Verification items for the finished model (mm, model axes). Give positions to 0.01 mm unless a question says otherwise; leave off trailing zeros. Order: outer loops, then holes, each group sorted by start corner. A loop starts at its lowest first (then second) coordinate and runs counter-clockwise, first axis right, second up.
(1) Sectioned sample at C-C on x = 76.2. Record the cut outline in (y, z) (3 decimals).
(2) Sectioned sample at B-B on z = 3.75. Count the separate pieces of the cut face and the enclosed holes in it, plus the area to 3 significant figures.
(3) Gauge pin test, flat end, axial feed: pin 1 (1 mm diameter, centred on y = -33, z = 4, fed in from +X). Record the tip position at first contact, or that the pin passes through.
(4) Sectioned sample at A-A on y = -32. Record the cut outline in (x, z), plus the area to 3 significant figures.
(5) Sectioned sample at D-D on y = -4.5. Record the cut outline in (x, z), plus the area to 3 significant figures.
(6) Scan lines: L1, parallel to Y at x = 0, z = 3; L2, parallel to X at y = -29.5, z = 4; L3, parallel to X at y = -9, z = 1. Record each from-to range of solid material in increasing order.
```python
from build123d import *

# Parameters (mm, degrees)
F0_R     = 1.5875
F1_DEPTH = 6.35


with BuildPart() as f1:
    # F0 (on Top) → F1 (new body)
    with BuildSketch(Plane.XY):
        with BuildLine():
            Line((152.4, 0), (0, 0))
            ThreePointArc((0, 0), (-19.05, -19.05), (0, -38.1))
            Line((0, -38.1), (60.325, -38.1))
            ThreePointArc((60.325, -38.1), (76.2, -22.225), (92.075, -38.1))
            Line((92.075, -38.1), (152.4, -38.1))
            ThreePointArc((152.4, -38.1), (171.45, -19.05), (152.4, 0))
        make_face()
        with Locations((0, -28.575)):
            Circle(F0_R, mode=Mode.SUBTRACT)
        with Locations((152.4, -28.575)):
            Circle(F0_R, mode=Mode.SUBTRACT)
        with Locations((0, -9.525)):
            Circle(F0_R, mode=Mode.SUBTRACT)
        with Locations((152.4, -9.525)):
            Circle(F0_R, mode=Mode.SUBTRACT)
    extrude(amount=F1_DEPTH)


solid = f1.part
```
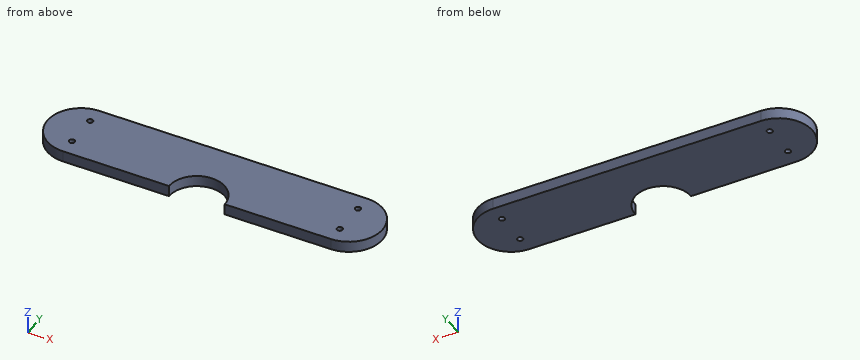
Ans:
1. outline: (-22.225, 0) - (0, 0) - (0, 6.35) - (-22.225, 6.35) - close
2. separate pieces: 1
2. enclosed holes: 4
2. area: 6,520 mm2
3. pin 1: stops at x = 165.89
4. outline: (-13.97, 0) - (61.54, 0) - (61.54, 6.35) - (-13.97, 6.35) - close; (90.86, 0) - (166.37, 0) - (166.37, 6.35) - (90.86, 6.35) - close
4. area: 959 mm2
5. outline: (-12.3, 0) - (164.7, 0) - (164.7, 6.35) - (-12.3, 6.35) - close
5. area: 1,120 mm2
6. L1: y = -38.1 to -30.16, -26.99 to -11.11, -7.94 to 0
6. L2: x = -15.93 to -1.29, 1.29 to 62.86, 89.54 to 151.11, 153.69 to 168.33
6. L3: x = -16.18 to -1.5, 1.5 to 150.9, 153.9 to 168.58
